Read the model definition and answer for the solid it produces. Units are mm, in the model's axes. A direction names the side the tool comes from. Coordinates: 2 decimals unless noted, no trailing zeros. Write each loop counter-clockwise with the first axis right and the second up, starting at its lowest first coordinate (ties: lowest second). Pieces come first, ordered by that corner, then holes. Notation, with made-up numbers: (28.25, -17) - (38.25, -17) arc R35 ccw to (38.25, 22) - close; hole circle Ø1 at (58, 68). An arc over 180 degrees is marked (long way). Use a Markdown table: item, result.
from build123d import *

# Parameters (mm, degrees)
SKETCH_W                                   = 15
SKETCH_H                                   = 36
PAD_DEPTH                                  = 6
SKETCH001_W                                = 20
SKETCH001_H                                = 3
POCKET_DEPTH                               = 2
SKETCH002_W                                = 3
SKETCH002_H                                = 3
POCKET001_DEPTH                            = 6.001
SKETCH003_R                                = 11
POCKET002_DEPTH                            = 36.001
SKETCH004_R                                = 1.65
POCKET003_DEPTH                            = 6.001
SKETCH005_R                                = 3.2
POCKET004_DEPTH                            = 4.001
CHAMFER004013007011015006009007001023_SIZE = 0.4
CHAMFER004013007011015006009007001024_SIZE = 1


with BuildPart() as part:
    # Sketch → Pad (new body)
    with BuildSketch(Plane.XY):
        Rectangle(SKETCH_W, SKETCH_H)
    extrude(amount=PAD_DEPTH)

    # Sketch001 (on Face5 of Pad) → Pocket (cut)
    with BuildSketch(Plane(origin=(0, 0, 0), x_dir=(1, 0, 0), z_dir=(0, 0, -1))):
        with Locations((0, 14.5)):
            Rectangle(SKETCH001_W, SKETCH001_H)
        with Locations((0, 4.5)):
            Rectangle(SKETCH001_W, SKETCH001_H)
        with Locations((0, -5.5)):
            Rectangle(SKETCH001_W, SKETCH001_H)
        with Locations((0, -14.5)):
            Rectangle(SKETCH001_W, SKETCH001_H)
    extrude(amount=-POCKET_DEPTH, mode=Mode.SUBTRACT)

    # Sketch002 (on Face10 of Pocket) → Pocket001 (cut, through all)
    with BuildSketch(Plane(origin=(0, 0, 0), x_dir=(1, 0, 0), z_dir=(0, 0, -1))):
        with Locations((-6.5, 14.5)):
            Rectangle(SKETCH002_W, SKETCH002_H)
        with Locations((6.5, 14.5)):
            Rectangle(SKETCH002_W, SKETCH002_H)
        with Locations((-6.5, 4.5)):
            Rectangle(SKETCH002_W, SKETCH002_H)
        with Locations((6.5, 4.5)):
            Rectangle(SKETCH002_W, SKETCH002_H)
        with Locations((-6.5, -5.5)):
            Rectangle(SKETCH002_W, SKETCH002_H)
        with Locations((6.5, -5.5)):
            Rectangle(SKETCH002_W, SKETCH002_H)
        with Locations((-6.5, -14.5)):
            Rectangle(SKETCH002_W, SKETCH002_H)
        with Locations((6.5, -14.5)):
            Rectangle(SKETCH002_W, SKETCH002_H)
    extrude(amount=-POCKET001_DEPTH, mode=Mode.SUBTRACT)

    # Sketch003 (on Face26 of Pocket001) → Pocket002 (cut, through all)
    with BuildSketch(Plane.XZ.offset(18)):
        with Locations((0, 15)):
            Circle(SKETCH003_R)
    extrude(amount=-POCKET002_DEPTH, mode=Mode.SUBTRACT)

    # Sketch004 (on Face77 of Pocket002) → Pocket003 (cut, through all)
    with BuildSketch(Plane(origin=(0, 0, 0), x_dir=(1, 0, 0), z_dir=(0, 0, -1))):
        with Locations((0, 9.5)):
            Circle(SKETCH004_R)
        with Locations((0, -10)):
            Circle(SKETCH004_R)
    extrude(amount=-POCKET003_DEPTH, mode=Mode.SUBTRACT)

    # Sketch005 (on Face74 of Pocket003) → Pocket004 (cut, through all)
    with BuildSketch(Plane(origin=(0, 0, 2), x_dir=(1, 0, 0), z_dir=(0, 0, -1))):
        with Locations((0, 9.5)):
            Circle(SKETCH005_R)
        with Locations((0, -10)):
            Circle(SKETCH005_R)
    extrude(amount=-POCKET004_DEPTH, mode=Mode.SUBTRACT)

    # Chamfer004013007011015006009007001023
    chamfer004013007011015006009007001023_edges = [part.edges().sort_by_distance(p)[0] for p in [
        (0, -18, 0),
        (-7.5, -18, 3),
        (-6.912278, -18, 6),
        (0, -18, 4),
        (6.912278, -18, 6),
        (7.5, -18, 3),
        (-7.5, -13, 1),
        (-7.5, -9.5, 0),
        (-7.5, -6, 1),
        (-7.5, -6, 4),
        (-7.5, -9.5, 6),
        (-7.5, -13, 4),
        (-7.5, -3, 4),
        (-7.5, -3, 1),
        (-7.5, 0.5, 0),
        (-7.5, 4, 1),
        (-7.5, 4, 4),
        (-7.5, 0.5, 6),
        (-7.5, 7, 4),
        (-7.5, 7, 1),
        (-7.5, 10, 0),
        (-7.5, 13, 1),
        (-7.5, 13, 4),
        (-7.5, 10, 6),
        (-7.5, 16, 4),
        (-7.5, 16, 1),
        (-7.5, 17, 0),
        (-7.5, 18, 3),
        (-7.5, 17, 6),
        (0, 18, 0),
        (7.5, 18, 3),
        (6.912278, 18, 6),
        (0, 18, 4),
        (-6.912278, 18, 6),
        (7.5, -16, 4),
        (7.5, -16, 1),
        (7.5, -17, 0),
        (7.5, -17, 6),
        (7.5, -6, 4),
        (7.5, -6, 1),
        (7.5, -9.5, 0),
        (7.5, -13, 1),
        (7.5, -13, 4),
        (7.5, -9.5, 6),
        (7.5, 4, 4),
        (7.5, 4, 1),
        (7.5, 0.5, 0),
        (7.5, -3, 1),
        (7.5, -3, 4),
        (7.5, 0.5, 6),
        (7.5, 13, 1),
        (7.5, 10, 0),
        (7.5, 7, 1),
        (7.5, 7, 4),
        (7.5, 10, 6),
        (7.5, 13, 4),
        (7.5, 17, 0),
        (7.5, 16, 1),
        (7.5, 16, 4),
        (7.5, 17, 6),
    ]]
    chamfer(chamfer004013007011015006009007001023_edges, length=CHAMFER004013007011015006009007001023_SIZE)

    # Chamfer004013007011015006009007001024
    chamfer004013007011015006009007001024_edges = [part.edges().sort_by_distance(p)[0] for p in [
        (-5, -14.5, 2),
        (5, -14.5, 2),
        (5, -4.5, 2),
        (-5, -4.5, 2),
        (-5, 5.5, 2),
        (5, 5.5, 2),
        (5, 14.5, 2),
        (-5, 14.5, 2),
    ]]
    chamfer(chamfer004013007011015006009007001024_edges, length=CHAMFER004013007011015006009007001024_SIZE)


solid = part.part
(1) A cutting plane is placed at A-A, the plane y = -9.5. Write down the section's boundary in (x, z).
Report:
| item | result |
|---|---|
| outline | (-7.5, 0.4) - (-7.1, 0) - (-1.65, 0) - (-1.65, 2) - (-3.2, 2) - (-3.2, 4.48) arc R11 cw to (-6.32, 6) - (-7.1, 6) - (-7.5, 5.6) - close; (1.65, 0) - (7.1, 0) - (7.5, 0.4) - (7.5, 5.6) - (7.1, 6) - (6.32, 6) arc R11 cw to (3.2, 4.48) - (3.2, 2) - (1.65, 2) - close |
(2) Each of these flat-tipped pins is pushed along its axis until it touches: P1, Ø8.5, axis at x = 0, y = 10, coming from the +Z side; P2, Ø3, axis at x = 0, y = -9.5, coming from the -Z side; P3, Ø1.8, axis at y = -4.5, z = 3.5, coming from the +X side; P4, Ø3, axis at x = 1.5, y = 9.5, coming from the +Z side. Where does it stop, or does it pass through?
Report:
| item | result |
|---|---|
| P1 | stops at z = 4.85 |
| P2 | passes through |
| P3 | stops at x = 5 |
| P4 | stops at z = 2 |
(3) The mould has two halves that part along X. Classify faces 4 (the flat face through (1.4, 8.6, 2)), 5 (the flat face through (0, 5, 2)), 6 (the flat face through (-4.5, -4.5, 2.5)), 7 (the conical face through (-0.1, 17.71, 3.89)): pulls with the +X half, pulls with the -X half, needs draft (parallel to the pull), parting line crosses it, or undercut.
Report:
| item | result |
|---|---|
| face 4 | undercut |
| face 5 | needs draft |
| face 6 | pulls with the -X half |
| face 7 | undercut |
(4) Straight lines are drawn through the part: L1, parallel to Y at x = 0, z = 3.3; L2, parallel to Y at x = 5.75, z = 1.5; L3, parallel to Y at x = 0, z = 3.7. For each, find the intervals that lie inside material, in ascending order.
Report:
| item | result |
|---|---|
| L1 | y = -18 to -12.7, -6.3 to 6.8, 13.2 to 18 |
| L2 | y = -18 to -16, -13 to -6, -3 to 4, 7 to 13, 16 to 18 |
| L3 | y = -17.9 to -12.7, -6.3 to 6.8, 13.2 to 17.9 |
(5) A cutting plane is placed at D-D, the plane y = 5.5. Write down the section's boundary in (x, z), and give its area (3 significant figures).
Report:
| item | result |
|---|---|
| outline | (-5, 3) - (-4, 2) - (4, 2) - (5, 3) - (5, 5.2) arc R11 cw to (-5, 5.2) - close |
| area | 22.9 mm² |
(6) For faces 1 (the flat face through (5, -4, 4)), 2 (the flat face through (-5, 15, 4)), 3 (the flat face through (4.5, -14.5, 2.5)), determine the directions among +Z, -Z, +X, -X, +Y, -Y from which every point of the face is accessible in a straight line to the end or side of a thin tool.
Report:
| item | result |
|---|---|
| face 1 | +Z, -Z, +X |
| face 2 | +Z, -Z, -X |
| face 3 | -Z, +X |
(7) A cutting plane is placed at B-B, the plane z = 1.25. Count the separate pieces of the cut face and the enclosed holes in it, and give its area (3 significant figures).
Report:
| item | result |
|---|---|
| separate pieces | 5 |
| enclosed holes | 2 |
| area | 341 mm² |
